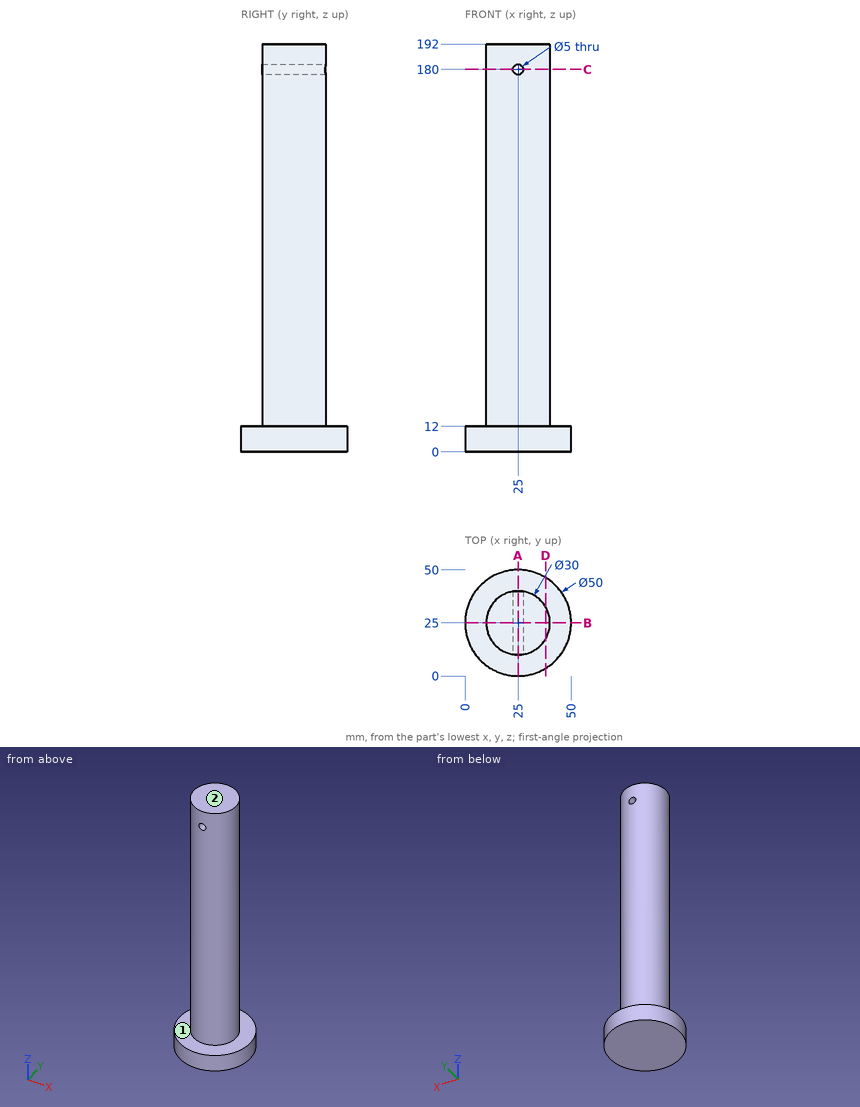
Could you check a few things on this drawing? It's one solid part, dimensions in mm from its lowest x, y, z. A direction names the side the tool comes from. Round coordinates to 2 decimals unless told otherwise and drop trailing zeros. Write each loop counter-clockwise with the first axis right and the second up, starting at its lowest first coordinate (ties: lowest second). Pieces come first, ordered by that corner, then holes.
Q1. If we section it at A-A on x = 25: Write out the boundary of the cut face in (y, z).
Q2. Please list where these lines run through material, in increasing order: probe 1 along Z at (x, y) = (25, 20); probe 2 along Z at (x, y) = (5, 36); probe 3 along X at (y, z) = (33.5, 180).
Q3. Which directions (+Z, -Z, +X, -X, +Y, -Y) give clear straight access to the entire face, cutting with the end or side of a thin tool? Please do the marked faces 1 and 2.
Q4. If we section it at B-B on y = 25: Write out the boundary of the cut face in (x, z).
Q5. If we section it at D-D on x = 38: Write out the boundary of the cut face in (y, z), plus the area to 3 significant figures.
Q6. If we section it at C-C on z = 180: Write out the boundary of the cut face in (x, y), plus the area to 3 significant figures.
Q7. Will these pins go through, and if not, where does the flat tip stop? P1, Ø1, axis at y = 22.5, z = 64.5, coming from the +X side; P2, Ø8, axis at x = 25, z = 180, coming from the -Y side; P3, Ø2, axis at x = 38, z = 156.5, coming from the +Y side.
Answer below:
1. outline: (0, 0) - (50, 0) - (50, 12) - (40, 12) - (40, 177.5) - (10, 177.5) - (10, 12) - (0, 12) - close; (10, 182.5) - (40, 182.5) - (40, 192) - (10, 192) - close
2. probe 1: z = 0 to 177.5, 182.5 to 192
2. probe 2: z = 0 to 12
2. probe 3: x = 12.64 to 22.5, 27.5 to 37.36
3. face 1: +Z
3. face 2: +Z, +X, -X, +Y, -Y
4. outline: (0, 0) - (50, 0) - (50, 12) - (40, 12) - (40, 192) - (10, 192) - (10, 12) - (0, 12) - close; hole circle Ø5 at (25, 180)
5. outline: (3.65, 0) - (46.35, 0) - (46.35, 12) - (32.48, 12) - (32.48, 192) - (17.52, 192) - (17.52, 12) - (3.65, 12) - close
5. area: 3,210 mm2
6. outline: (22.5, 10.21) - (22.5, 39.79) arc R15 ccw to start; (27.5, 10.21) arc R15 ccw to (27.5, 39.79) - close
6. area: 558 mm2
7. P1: stops at x = 39.87
7. P2: stops at y = 10
7. P3: stops at y = 34
